from build123d import *

# Parameters (mm, degrees)
SKETCH2_R           = 9
SKETCH2_R_2         = 2.05
SKETCH2_R_3         = 1.575
BOSS_EXTRUDE2_DEPTH = 4.7
BOSS_EXTRUDE3_START = -4.7
BOSS_EXTRUDE3_DEPTH = 4.7
FILLET1_R           = 0.5


with BuildPart() as part:
    # Sketch2 → Boss-Extrude2 (new body)
    with BuildSketch(Plane(origin=(0, 0, 0), x_dir=(1, 0, 0), z_dir=(0, 1, 0))):
        with Locations(Location((0, 0, 0), (0, 0, 270))):
            Circle(SKETCH2_R)
        with Locations(Location((0, 0, 0), (0, 0, 270))):
            Circle(SKETCH2_R_2, mode=Mode.SUBTRACT)
        with Locations(Location((-4.242640687, 4.242640687, 0), (0, 0, 270))):
            Circle(SKETCH2_R_3, mode=Mode.SUBTRACT)
        with Locations(Location((-4.242640687, -4.242640687, 0), (0, 0, 270))):
            Circle(SKETCH2_R_3, mode=Mode.SUBTRACT)
        with Locations(Location((4.242640687, -4.242640687, 0), (0, 0, 270))):
            Circle(SKETCH2_R_3, mode=Mode.SUBTRACT)
        with Locations(Location((4.242640687, 4.242640687, 0), (0, 0, 270))):
            Circle(SKETCH2_R_3, mode=Mode.SUBTRACT)
    extrude(amount=BOSS_EXTRUDE2_DEPTH)

    # Sketch3 → Boss-Extrude3 (add)
    with BuildSketch(Plane(origin=(0, 4.7, 0), x_dir=(1, 0, 0), z_dir=(0, 1, 0)).offset(BOSS_EXTRUDE3_START)):
        with BuildLine():
            Line((-2, 35.606375805), (-2, 8.774964387))
            ThreePointArc((-2, 8.774964387), (0, 9), (2, 8.774964387))
            Line((2, 8.774964387), (2, 35.606375805))
            Line((2, 35.606375805), (4.264997114, 35.606375805))
            Line((4.264997114, 35.606375805), (0, 42))
            Line((0, 42), (-4.264997114, 35.606375805))
            Line((-4.264997114, 35.606375805), (-2, 35.606375805))
        make_face()
    extrude(amount=BOSS_EXTRUDE3_DEPTH)

    # Fillet1
    fillet1_edges = [part.edges().sort_by_distance(p)[0] for p in [
        (-3.132498557, 4.7, -35.606375805),
        (-2, 4.7, -22.190670096),
        (2, 4.7, -22.190670096),
        (3.132498557, 4.7, -35.606375805),
        (2.132498557, 4.7, -38.803187903),
        (-2.132498557, 4.7, -38.803187903),
        (-3.132498557, 0, -35.606375805),
        (-2.132498557, 0, -38.803187903),
        (2.132498557, 0, -38.803187903),
        (3.132498557, 0, -35.606375805),
        (2, 0, -22.190670096),
        (-2, 0, -22.190670096),
    ]]
    fillet(fillet1_edges, radius=FILLET1_R)


solid = part.part
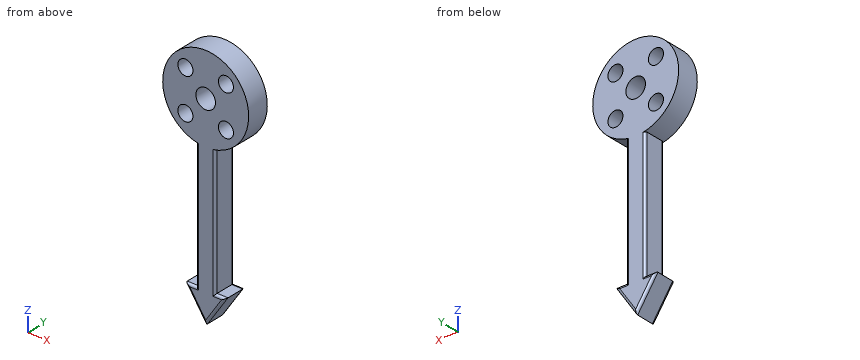
Here's how the part is built. I have some questions about the finished solid (model axes, mm). Round coordinates to 2 decimals unless told otherwise and drop trailing zeros. Loops run counter-clockwise (first coordinate to the right, second up) from the corner with the lowest first, then second, coordinate; pieces in that order, holes last. Notation, with made-up numbers: M 80,61.25 L 90,61.25 A31 ccw 90,92.25 Z; hole C -39.75,14.25 d1. An arc over 180 degrees is marked long. Write each question's results on one line, items separated by ' | '. Start each with the question number.
(1) Will these pins go through, and if not, where does the flat tip stop? P1, Ø1, axis at y = 3.5, z = -8, coming from the -X side; P2, Ø2.5, axis at x = 3, y = 1.5, coming from the +Z side; P3, Ø1.8, axis at y = 3, z = -17, coming from the -X side.
(2) If I drill on probe 1 along Z at (x, y) = (4.75, 1.8); probe 2 along X at (y, z) = (2.65, 3.5); probe 3 along Z at (x, y) = (-3.5, 1), over which ranges is the centre line in solid material (lowest first)? Write a range as from..to.
(3) I want a section at C-C (y = 1.5). Please give me the cut outline in (x, z) (3 decimals), then the cut area to 3 significant figures.
(4) I want a section at B-B (z = -16.5). Please give me the cut outline in (x, y).
(5) I want a section at A-A (z = 0). Please give me the cut outline in (x, y).
Solved:
1) P1: stops at x = -4.97 | P2: stops at z = 8.83 | P3: stops at x = -2
2) probe 1: z = -7.64..-5.73, -2.75..2.75, 5.73..7.64 | probe 2: x = -8.29..-5.63, -2.85..2.85, 5.63..8.29 | probe 3: z = -36.75..-35.61, -8.29..-5.63, -2.85..2.85, 5.63..8.29
3) outline: M -4.265,-35.606 L 0,-42 L 4.265,-35.606 L 2,-35.606 L 2,-8.775 A9 ccw long -2,-8.775 L -2,-35.606 Z; hole C -4.243,-4.243 d3.15; hole C -4.243,4.243 d3.15; hole C 0,0 d4.1; hole C 4.243,-4.243 d3.15; hole C 4.243,4.243 d3.15 | area: 344 mm²
4) outline: M -2,0.5 A0.5 ccw -1.5,0 L 1.5,0 A0.5 ccw 2,0.5 L 2,4.2 A0.5 ccw 1.5,4.7 L -1.5,4.7 A0.5 ccw -2,4.2 Z
5) outline: M -9,0 L -2.05,0 L -2.05,4.7 L -9,4.7 Z; M 2.05,0 L 9,0 L 9,4.7 L 2.05,4.7 Z
